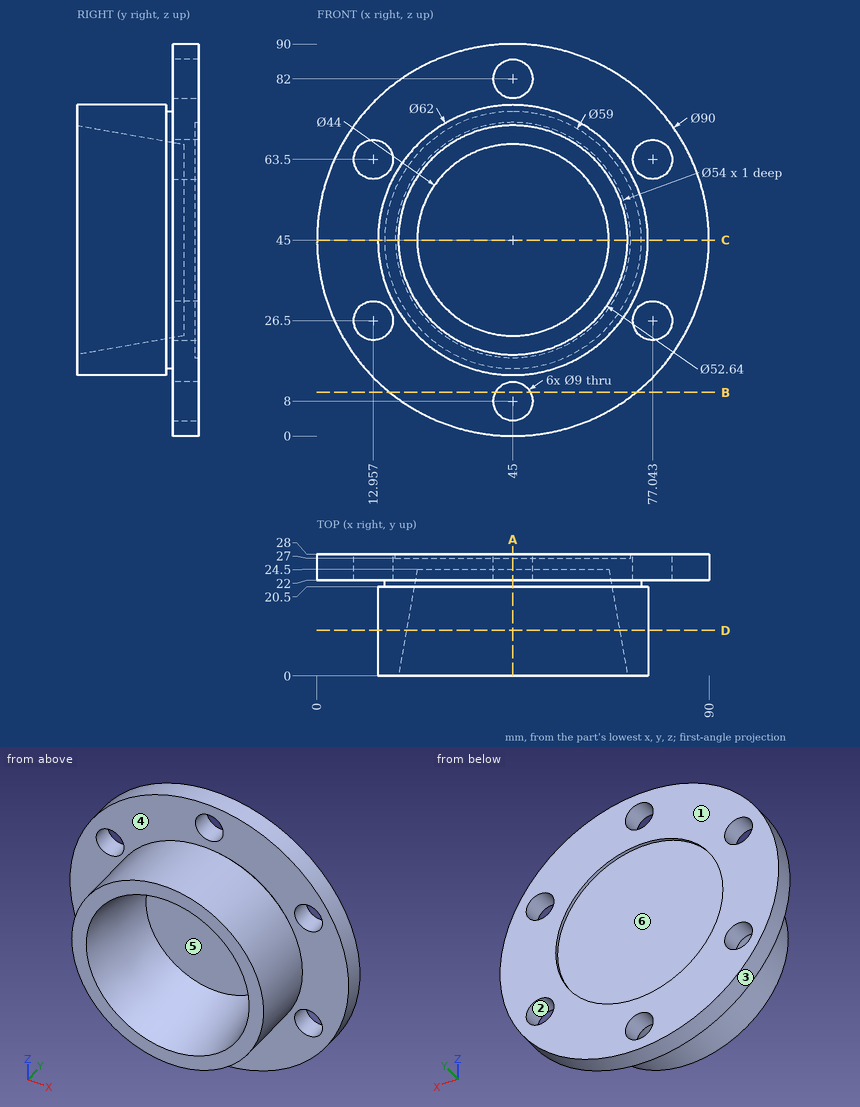
The figure shows three views and two pictorial views of one solid part (mm, origin at its lowest corner). Answer the questions. A direction names the side the tool comes from. Give positions to 0.01 mm unless a question says otherwise; leave off trailing zeros. Write each loop counter-clockwise with the first axis right and the second up, starting at its lowest first coordinate (ties: lowest second). Pieces come first, ordered by that corner, then holes. Notation, with made-up numbers: (34, 72) - (77, 72) arc R20 ccw to (77, 108) - close; hole circle Ø4 at (30.5, -28.5). An arc over 180 degrees is marked (long way). Use CSV: the item, a comma, the result in double quotes. Start each with the question number.
Item 1: The part is cut by section C-C, the plane z = 45. Give the vertices of the cut face in (x, y).
Item 2: The part is cut by section D-D, the plane y = 10.5. Give the vertices of the cut face in (x, z), and give its area (3 significant figures).
Item 3: The mould has two halves that part along X. Classify the marked faces 1, 2 and 3: pulls with the +X half, pulls with the -X half, needs draft (parallel to the pull), parting line crosses it, or undercut.
Item 4: For the marked faces 4, 5 and 6, determine the directions among +Z, -Z, +X, -X, +Y, -Y from which every point of the face is accessible in a straight line to the end or side of a thin tool.
Item 5: The part is cut by section A-A, the plane x = 45. Give the vertices of the cut face in (y, z).
Item 6: Flat-ended cylindrical pins translate along their axes: P1, Ø8, axis at x = 31, z = 80.5, coming from the -Y side; P2, Ø22, axis at x = 35.5, z = 40, coming from the -Y side; P3, Ø14.5, axis at x = 12.96, z = 26.5, coming from the -Y side; P4, Ø12, axis at x = 41.5, y = 8.5, coming from the -Z side. Find the tip coordinate at first contact, or state that the pin passes through.
Item 7: The part is cut by section B-B, the plane z = 10. Give the vertices of the cut face in (x, y).
Item 8: Consider line 1 (X direction, y = 26, z = 26.5); line 2 (X direction, y = 27.8, z = 45); line 3 (Z direction, x = 42, y = 25.5). Determine where each line is inside the solid, lowest interval first.
Taken from the geometry:
1,outline,"(0, 22) - (15.5, 22) - (15.5, 20.5) - (14, 20.5) - (14, 0) - (18.68, 0) - (23, 24.5) - (67, 24.5) - (71.32, 0) - (76, 0) - (76, 20.5) - (74.5, 20.5) - (74.5, 22) - (90, 22) - (90, 28) - (72, 28) - (72, 27) - (18, 27) - (18, 28) - (0, 28) - close"
2,outline,"circle Ø62 at (45, 45); hole circle Ø48.94 at (45, 45)"
2,area,"1,140 mm2"
3,face 1,"needs draft"
3,face 2,"undercut"
3,face 3,"parting line crosses it"
4,face 4,"none"
4,face 5,"-Y"
4,face 6,"+Y"
5,outline,"(0, 14) - (20.5, 14) - (20.5, 15.5) - (22, 15.5) - (22, 12.5) - (28, 12.5) - (28, 18) - (27, 18) - (27, 72) - (28, 72) - (28, 77.5) - (22, 77.5) - (22, 74.5) - (20.5, 74.5) - (20.5, 76) - (0, 76) - (0, 71.32) - (24.5, 67) - (24.5, 23) - (0, 18.68) - close; (22, 0) - (28, 0) - (28, 3.5) - (22, 3.5) - close; (22, 86.5) - (28, 86.5) - (28, 90) - (22, 90) - close"
6,P1,"y = 22"
6,P2,"y = 24.5"
6,P3,"y = 0"
6,P4,"z = 14"
7,outline,"(16.72, 22) - (40.97, 22) - (40.97, 28) - (16.72, 28) - close; (49.03, 22) - (73.28, 22) - (73.28, 28) - (49.03, 28) - close"
8,line 1,"3.98 to 8.46, 17.46 to 72.54, 81.54 to 86.02"
8,line 2,"0 to 18, 72 to 90"
8,line 3,"0.1 to 4.65, 11.35 to 78.65, 85.35 to 89.9"
